```python
from build123d import *

# Parameters (mm, degrees)
F0_W     = 100
F0_H     = 100
F0_W_2   = 85
F0_H_2   = 35
F0_W_3   = 80
F0_H_3   = 30
F1_DEPTH = 2
F2_DEPTH = 4
F3_W     = 85
F3_H     = 2
F4_DEPTH = 2
F5_W     = 85
F5_H     = 2
F6_DEPTH = 2
F7_DEPTH = 2
F8_W     = 30
F8_H     = 6
F9_DEPTH = 3.5


with BuildPart() as f1:
    # F0 (on Front) → F1 (new body)
    with BuildSketch(Plane.XZ):
        Rectangle(F0_W, F0_H)
        Rectangle(F0_W_2, F0_H_2, mode=Mode.SUBTRACT)
        Rectangle(F0_W_2, F0_H_2)
        Rectangle(F0_W_3, F0_H_3, mode=Mode.SUBTRACT)
        Rectangle(F0_W_3, F0_H_3)
    extrude(amount=-F1_DEPTH)

    # F0 (on Front) → F2 (join)
    with BuildSketch(Plane.XZ):
        Rectangle(F0_W_2, F0_H_2)
        Rectangle(F0_W_3, F0_H_3, mode=Mode.SUBTRACT)
    extrude(amount=F2_DEPTH)

    # F3 (on face) → F4 (join)
    with BuildSketch(Plane(origin=(0, 0, -17.5), x_dir=(1, 0, 0), z_dir=(0, 0, -1))):
        with Locations((0, 3)):
            Rectangle(F3_W, F3_H)
    extrude(amount=F4_DEPTH)

    # F5 (on face) → F6 (join)
    with BuildSketch(Plane.XY.offset(17.5)):
        with Locations((0, -3)):
            Rectangle(F5_W, F5_H)
    extrude(amount=F6_DEPTH)

    # F0 (on Front) → F7 (join)
    with BuildSketch(Plane.XZ):
        Rectangle(F0_W_3, F0_H_3)
    extrude(amount=F7_DEPTH)

    # F8 (on face) → F9 (cut)
    with BuildSketch(Plane(origin=(0, 2, 0), x_dir=(-1, 0, 0), z_dir=(0, 1, 0))):
        Rectangle(F8_W, F8_H)
    extrude(amount=-F9_DEPTH, mode=Mode.SUBTRACT)


solid = f1.part
```
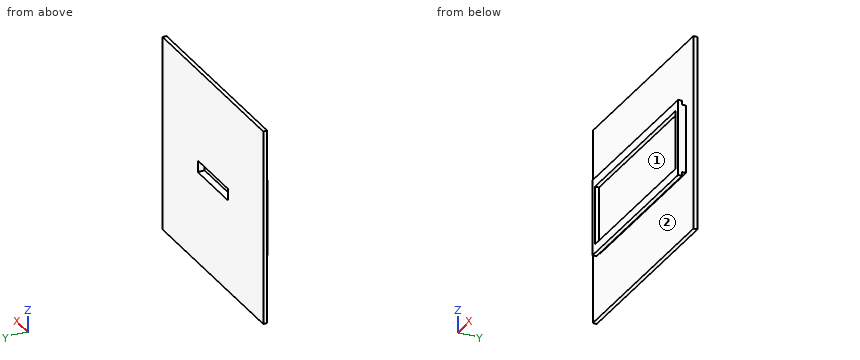
Can you work these out from the model? Positions are in its coordinate system, mm. Face numbers are marked on the shaded views. Give positions to 0.01 mm unless a question says otherwise; leave off trailing zeros. Loops run counter-clockwise (first coordinate to the right, second up) from the corner with the lowest first, then second, coordinate; pieces in that order, holes last. Notation, with made-up numbers: M 0.5,-14.5 L 58.5,-14.5 A13 ccw 58.5,3.5 Z; hole C 60.25,19.25 d4. An arc over 180 degrees is marked long. One line per question, with ' | ' between items. Start each with the question number.
Q1. If we section it at A-A (x = -38): Please give me the cut outline in (y, z), plus the area to 3 significant figures.
Q2. If we section it at D-D (z = 34): Please give me the cut outline in (x, y).
Q3. If we section it at B-B (z = 8.5): Please give me the cut outline in (x, y), plus the area to 3 significant figures.
Q4. If we mould it in two halves opening along X, with no side actions, what happens to the marked faces 1 and 2? For each: +X half, -X half, draft (parallel to the pull), parting line (faces both ways), or undercut.
Q5. For pin 1 Ø2 at (x, y) = (5.5, -2.5) entering from -Z; pin 2 Ø9 at (x, z) = (4, -7) entering from -Y; pin 3 Ø1 at (y, z) = (-3, -2) entering from +X, each with a flat end and sliding along its axis, tell me the tip position at first contact or that it passes through.
Q6. If we section it at C-C (x = -10.5): Please give me the cut outline in (y, z).
Q7. If I drill on line 1 (Z direction, x = 6.5, y = 1); line 2 (Z direction, x = -19, y = -2.7); line 3 (Y direction, x = 32, z = -18.5), over which ranges is the centre line in solid material (lowest first)? Write a range as from..to.
Computed:
1) outline: M -4,-19.5 L -2,-19.5 L -2,-17.5 L 0,-17.5 L 0,-50 L 2,-50 L 2,50 L 0,50 L 0,17.5 L -2,17.5 L -2,19.5 L -4,19.5 L -4,15 L -2,15 L -2,-15 L -4,-15 Z | area: 288 mm²
2) outline: M -50,0 L 50,0 L 50,2 L -50,2 Z
3) outline: M -50,0 L -42.5,0 L -42.5,-4 L -40,-4 L -40,-2 L 40,-2 L 40,-4 L 42.5,-4 L 42.5,0 L 50,0 L 50,2 L -50,2 Z | area: 380 mm²
4) face 1: undercut | face 2: draft
5) pin 1: stops at z = -19.5 | pin 2: stops at y = -2 | pin 3: stops at x = 42.5
6) outline: M -4,-19.5 L -2,-19.5 L -2,-17.5 L 0,-17.5 L 0,-50 L 2,-50 L 2,-3 L -1.5,-3 L -1.5,3 L 2,3 L 2,50 L 0,50 L 0,17.5 L -2,17.5 L -2,19.5 L -4,19.5 L -4,15 L -2,15 L -2,-15 L -4,-15 Z
7) line 1: z = -50..-3, 3..50 | line 2: z = -19.5..-15, 15..19.5 | line 3: y = -4..-2, 0..2
